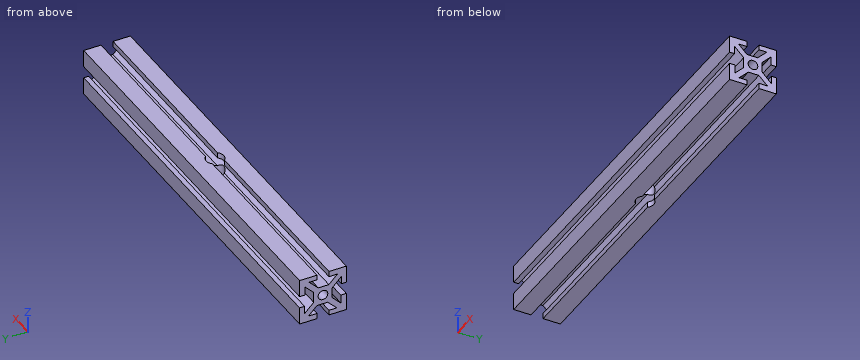
```python
from build123d import *

# Parameters (mm, degrees)
SKETCH1_W               = 10
SKETCH1_H               = 10
SKETCH1_R               = 2.605
BOSS_EXTRUDE1_DEPTH     = 215.9
CIRPATTERN1_COUNT       = 4
SKETCH2_R               = 4.765
CUT_EXTRUDE2_DEPTH      = 10
CUT_EXTRUDE2_DEPTH_BACK = 50


with BuildPart() as part:
    # Sketch1 → Boss-Extrude1 (new body)
    with BuildSketch(Plane(origin=(0, 0, 0), x_dir=(0, 0, -1), z_dir=(1, 0, 0))):
        Rectangle(SKETCH1_W, SKETCH1_H)
        Circle(SKETCH1_R, mode=Mode.SUBTRACT)
        Polygon((7.474873734, 9.921463197), (2.553410537, 5), (5, 5), (5, 3.203948776), (9.596194078, 7.800142853), align=None)
        Polygon((9.596194078, 3.24), (12.596194078, 3.24), (12.596194078, 12.596194078), (3.24, 12.596194078), (3.24, 9.921463197), (7.474873734, 9.921463197), (9.596194078, 7.800142853), align=None)
    boss_extrude1 = extrude(amount=BOSS_EXTRUDE1_DEPTH)

    # CirPattern1: Boss-Extrude1 ×4 about axis
    cirpattern1_axis = Axis((0, 0, 0), (1, 0, 0))
    for i in range(1, CIRPATTERN1_COUNT):
        add(boss_extrude1.rotate(cirpattern1_axis, i * 360 / CIRPATTERN1_COUNT))

    # Sketch2 → Cut-Extrude2 (cut, two sides)
    with BuildSketch(Plane.XY.offset(12.596194078)) as cut_extrude2_sk:
        with Locations((107.95, 0)):
            Circle(SKETCH2_R)
    extrude(amount=CUT_EXTRUDE2_DEPTH, mode=Mode.SUBTRACT)
    extrude(cut_extrude2_sk.sketch, amount=-CUT_EXTRUDE2_DEPTH_BACK, mode=Mode.SUBTRACT)


solid = part.part
```
Here's how the part is built. I have some questions about the finished solid (model axes, mm). Give positions to 0.01 mm unless a question says otherwise; leave off trailing zeros. Write each loop counter-clockwise with the first axis right and the second up, starting at its lowest first coordinate (ties: lowest second). Pieces come first, ordered by that corner, then holes. Notation, with made-up numbers: (4.5, -34.5) -> (54.5, -34.5) arc R10 cw to (54.5, -30.5) -> close; hole circle Ø3 at (12.5, -28). An arc over 180 degrees is marked (long way). Write each question's results on one line, items separated by ' | '.
Item 1: Suppose I cut it at A-A on y = 0. Write out the boundary of the cut face in (x, z) (3 decimals).
Output:
outline: (0, -5) -> (103.185, -5) -> (103.185, -2.605) -> (0, -2.605) -> close; (0, 2.605) -> (103.185, 2.605) -> (103.185, 5) -> (0, 5) -> close; (112.715, -5) -> (215.9, -5) -> (215.9, -2.605) -> (112.715, -2.605) -> close; (112.715, 2.605) -> (215.9, 2.605) -> (215.9, 5) -> (112.715, 5) -> close
Item 2: Suppose I cut it at B-B on z = 0. Write out the boundary of the cut face in (x, y) (3 decimals), plus the area to 3 significant figures.
Output:
outline: (0, -5) -> (215.9, -5) -> (215.9, -2.605) -> (111.94, -2.605) arc R4.765 cw to (103.96, -2.605) -> (0, -2.605) -> close; (0, 2.605) -> (103.96, 2.605) arc R4.765 cw to (111.94, 2.605) -> (215.9, 2.605) -> (215.9, 5) -> (0, 5) -> close | area: 1,010 mm^2
Item 3: If I drill on L1, parallel to Y at x = 28, z = 10; L2, parallel to Y at x = 45, z = 0 (3 decimals); L3, parallel to Y at x = 49, z = -5.25, over which ranges is the centre line in solid material (lowest first)?
Output:
L1: y = -12.6 to -3.24, 3.24 to 12.6 | L2: y = -5 to -2.605, 2.605 to 5 | L3: y = -12.6 to -9.6, -7.05 to -2.8, 3.45 to 7.7, 9.92 to 12.6
Item 4: For pin 1 Ø1.7 at (x, y) = (54.5, -1.5) entering from +Z; pin 2 Ø3 at (x, z) = (133, 1.5) entering from +Y; pin 3 Ø3 at (x, y) = (177.5, 1) entering from -Z, each with a flat end and sliding along its axis, tell me the tip position at first contact or that it passes through.
Output:
pin 1: stops at z = 5 | pin 2: stops at y = 5 | pin 3: stops at z = -5
